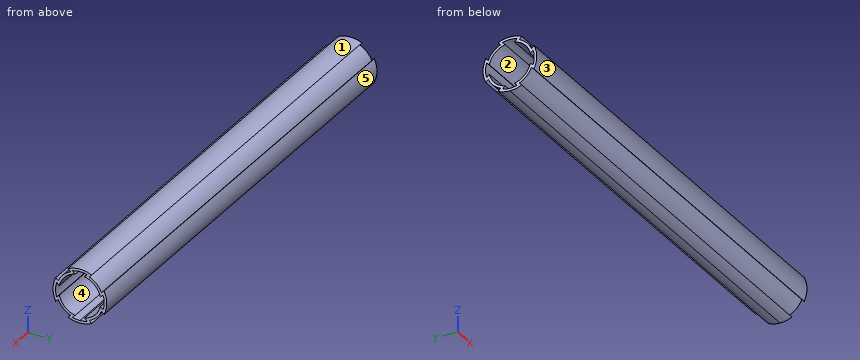
from build123d import *

# Parameters (mm, degrees)
BOSS_EXTRUDE1_DEPTH = 249


with BuildPart() as part:
    # Sketch1 → Boss-Extrude1 (new body)
    with BuildSketch(Plane(origin=(0, 0, 0), x_dir=(0, 0, -1), z_dir=(1, 0, 0))):
        with BuildLine():
            Line((-11.297790668, 4.86311896), (-12.579426967, 6.144755258))
            ThreePointArc((-12.579426967, 6.144755258), (-14, 0), (-12.579426967, -6.144755258))
            Line((-12.579426967, -6.144755258), (-11.297790668, -4.86311896))
            ThreePointArc((-11.297790668, -4.86311896), (-8.697413409, -8.697413409), (-4.86311896, -11.297790668))
            Line((-4.86311896, -11.297790668), (-6.144755258, -12.579426967))
            ThreePointArc((-6.144755258, -12.579426967), (0, -14), (6.144755258, -12.579426967))
            Line((6.144755258, -12.579426967), (4.86311896, -11.297790668))
            ThreePointArc((4.86311896, -11.297790668), (8.697413409, -8.697413409), (11.297790668, -4.86311896))
            Line((11.297790668, -4.86311896), (12.579426967, -6.144755258))
            ThreePointArc((12.579426967, -6.144755258), (13.64023419, -3.153412633), (14, 0))
            ThreePointArc((14, 0), (13.64023419, 3.153412633), (12.579426967, 6.144755258))
            Line((12.579426967, 6.144755258), (11.297790668, 4.86311896))
            ThreePointArc((11.297790668, 4.86311896), (8.697413409, 8.697413409), (4.86311896, 11.297790668))
            Line((4.86311896, 11.297790668), (6.144755258, 12.579426967))
            ThreePointArc((6.144755258, 12.579426967), (0, 14), (-6.144755258, 12.579426967))
            Line((-6.144755258, 12.579426967), (-4.86311896, 11.297790668))
            ThreePointArc((-4.86311896, 11.297790668), (-8.697413409, 8.697413409), (-11.297790668, 4.86311896))
        make_face()
        with BuildLine():
            Line((-10.723588409, 2.450439069), (-12.107380777, 3.834231437))
            ThreePointArc((-12.107380777, 3.834231437), (-12.7, 0), (-12.107380777, -3.834231437))
            Line((-12.107380777, -3.834231437), (-10.723588409, -2.450439069))
            ThreePointArc((-10.723588409, -2.450439069), (-7.778174593, -7.778174593), (-2.450439069, -10.723588409))
            Line((-2.450439069, -10.723588409), (-3.834231437, -12.107380777))
            ThreePointArc((-3.834231437, -12.107380777), (0, -12.7), (3.834231437, -12.107380777))
            Line((3.834231437, -12.107380777), (2.450439069, -10.723588409))
            ThreePointArc((2.450439069, -10.723588409), (7.778174593, -7.778174593), (10.723588409, -2.450439069))
            Line((10.723588409, -2.450439069), (12.107380777, -3.834231437))
            ThreePointArc((12.107380777, -3.834231437), (12.550970797, -1.939879394), (12.7, 0))
            ThreePointArc((12.7, 0), (12.550970797, 1.939879394), (12.107380777, 3.834231437))
            Line((12.107380777, 3.834231437), (10.723588409, 2.450439069))
            ThreePointArc((10.723588409, 2.450439069), (7.778174593, 7.778174593), (2.450439069, 10.723588409))
            Line((2.450439069, 10.723588409), (3.834231437, 12.107380777))
            ThreePointArc((3.834231437, 12.107380777), (0, 12.7), (-3.834231437, 12.107380777))
            Line((-3.834231437, 12.107380777), (-2.450439069, 10.723588409))
            ThreePointArc((-2.450439069, 10.723588409), (-7.778174593, 7.778174593), (-10.723588409, 2.450439069))
        make_face(mode=Mode.SUBTRACT)
    extrude(amount=BOSS_EXTRUDE1_DEPTH)


solid = part.part
Build history of the part. All positions in model axes, mm. Face numbers are marked on the shaded views. A direction names the side the tool comes from. Round coordinates to 2 decimals unless told otherwise and drop trailing zeros. Write each loop counter-clockwise with the first axis right and the second up, starting at its lowest first coordinate (ties: lowest second). Pieces come first, ordered by that corner, then holes. Notation, with made-up numbers: M -33,32.5 L 2,32.5 A24 ccw 2,48.5 Z; hole C 84.5,-17.5 d3. An arc over 180 degrees is marked long. Use CSV: the item, a comma, the result in double quotes.
1. Saw through at A-A (z = 8.5). Give the cut face in (x, y), plus the area to 3 significant figures.
Reply:
outline,"M 0,-8.89 L 249,-8.89 L 249,-6.98 L 0,-6.98 Z; M 0,6.98 L 249,6.98 L 249,8.89 L 0,8.89 Z"
area,"950 mm²"
2. Tool access for the marked faces 4 and 5: list every direction of +Z, -Z, +X, -X, +Y, -Y with a clear straight run to the whole face (end or side of a thin tool).
Reply:
face 4,"+X, -X"
face 5,"+X, -X, +Y"
3. Two-plate mould, pull along Z, no slides. Class the marked faces 1, 2 and 3: +Z half, -Z half, draft (parallel to the pull), parting line (faces both ways), or undercut.
Reply:
face 1,"+Z half"
face 2,"undercut"
face 3,"parting line"
4. Flat gauge pins, fed straight in: pin 1 (1 mm diameter, centred on x = 64.5, y = 8.5, fed in from +Z); pin 2 (5 mm diameter, centred on x = 109.5, z = 6.5, fed in from -Y); pin 3 (8 mm diameter, centred on x = 98, y = 8, fed in from +Z); pin 4 (2 mm diameter, centred on y = -10, z = -10.5, fed in from +X). Where does each tip first touch, or does it go through?
Reply:
pin 1,"stops at z = 9.34"
pin 2,"stops at y = -13.42"
pin 3,"stops at z = 13.42"
pin 4,"passes through"
5. Wall check: probe 1 along Y at (x, z) = (201.5, 5.5); probe 2 along Z at (x, y) = (38.5, -0.75); probe 3 along Z at (x, y) = (212, 5.25). Give the ranges that are in metal, low to high. Write a range as from..to.
Reply:
probe 1,"y = -12.87..-11.93, -11..-9.53, 9.53..11, 11.93..12.87"
probe 2,"z = -13.98..-12.68, 12.68..13.98"
probe 3,"z = -12.98..-11.68, -11.12..-9.67, 9.67..11.12, 11.68..12.98"
